The figure shows three views and two pictorial views of one solid part (mm, origin at its lowest corner). Answer the questions. A direction names the side the tool comes from. Give positions to 0.01 mm unless a question says otherwise; leave off trailing zeros. Write each loop counter-clockwise with the first axis right and the second up, starting at its lowest first coordinate (ties: lowest second). Pieces come first, ordered by that corner, then holes. Notation, with made-up numbers: (72.5, 45) -> (110.5, 45) arc R31 ccw to (110.5, 75) -> close; hole circle Ø10 at (25.5, 50.25). An arc over 180 degrees is marked (long way). Use a Markdown table: item, result.
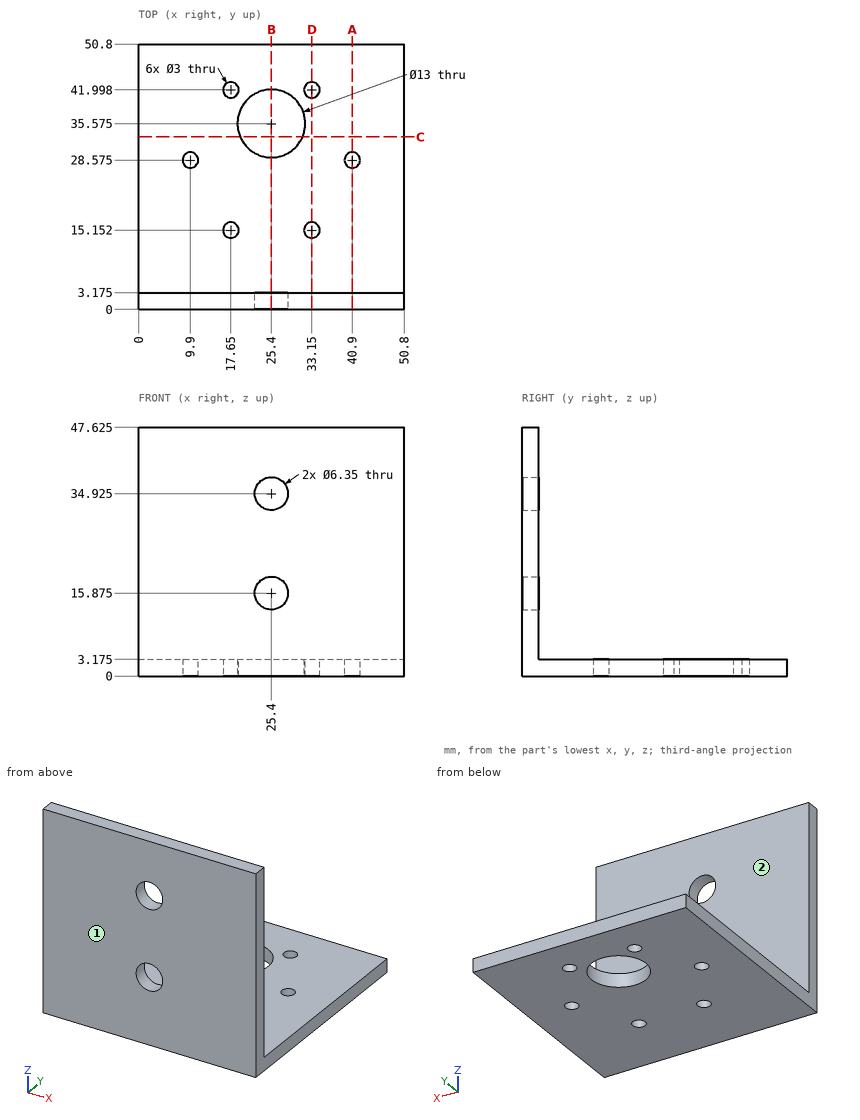
Item 1: Straight lines are drawn through the part: line 1 along Y through (x, z) = (40.9, 1.7) (1 decimal); line 2 along Z through (x, y) = (13, 15) (1 decimal). For each, find the intervals that lie inside material, in ascending order. Write a range as [from, to].
Return value:
| item | result |
|---|---|
| line 1 | [0, 27.1], [30.1, 50.8] |
| line 2 | [0, 3.2] |
Item 2: A tool of negligible diameter and unlimited length cuts with its end or side. For the marked faces 1 and 2, from which of +Z, -Z, +X, -X, +Y, -Y can it reach the whole face along a straight path? Write none if from no direction.
Return value:
| item | result |
|---|---|
| face 1 | +Z, -Z, +X, -X, -Y |
| face 2 | +Z, +X, -X, +Y |
Item 3: A cutting plane is placed at C-C (y = 33). Give the vertices of the cut face in (x, z) (1 decimal), then the cut area to 3 significant figures.
Return value:
| item | result |
|---|---|
| outline | (0, 0) -> (19.4, 0) -> (19.4, 3.2) -> (0, 3.2) -> close; (31.4, 0) -> (50.8, 0) -> (50.8, 3.2) -> (31.4, 3.2) -> close |
| area | 123 mm^2 |
Item 4: Each of these flat-tipped pins is pushed along its axis until it touches: P1, Ø6, axis at x = 45, z = 27.5, coming from the +Y side (3 decimals); P2, Ø3, axis at x = 25, y = 12.5, coming from the +Z side (3 decimals). Where does it stop, or does it pass through?
Return value:
| item | result |
|---|---|
| P1 | y = 3.175 |
| P2 | z = 3.175 |
Item 5: A cutting plane is placed at A-A (x = 40.9). Give the vertices of the cut face in (y, z) (1 decimal).
Return value:
| item | result |
|---|---|
| outline | (0, 0) -> (27.1, 0) -> (27.1, 3.2) -> (3.2, 3.2) -> (3.2, 47.6) -> (0, 47.6) -> close; (30.1, 0) -> (50.8, 0) -> (50.8, 3.2) -> (30.1, 3.2) -> close |
Item 6: A cutting plane is placed at D-D (x = 33.15). Give the vertices of the cut face in (y, z) (1 decimal).
Return value:
| item | result |
|---|---|
| outline | (0, 0) -> (13.7, 0) -> (13.7, 3.2) -> (3.2, 3.2) -> (3.2, 47.6) -> (0, 47.6) -> close; (16.7, 0) -> (40.5, 0) -> (40.5, 3.2) -> (16.7, 3.2) -> close; (43.5, 0) -> (50.8, 0) -> (50.8, 3.2) -> (43.5, 3.2) -> close |
Item 7: A cutting plane is placed at B-B (x = 25.4). Count the separate pieces of the cut face and the enclosed holes in it, then the cut area to 3 significant figures.
Return value:
| item | result |
|---|---|
| separate pieces | 4 |
| enclosed holes | 0 |
| area | 221 mm^2 |
